from build123d import *

# Parameters (mm, degrees)
SKETCH3_W           = 152.4
SKETCH3_H           = 152.4
BOSS_EXTRUDE1_DEPTH = 12.7
SKETCH5_W           = 147.32
SKETCH5_H           = 7.62
CUT_EXTRUDE1_DEPTH  = 12.7
SKETCH6_W           = 12.7
SKETCH6_H           = 127
CUT_EXTRUDE3_DEPTH  = 12.7
SKETCH8_W           = 7.62
SKETCH8_H           = 7.62
CUT_EXTRUDE4_DEPTH  = 25.4
SKETCH9_W           = 7.62
SKETCH9_H           = 7.62
CUT_EXTRUDE5_DEPTH  = 25.4
SKETCH10_W          = 7.508888552
SKETCH10_H          = 7.62
CUT_EXTRUDE6_DEPTH  = 25.4
SKETCH11_W          = 7.62
SKETCH11_H          = 7.62
BOSS_EXTRUDE3_DEPTH = 25.4
SKETCH12_W          = 7.62
SKETCH12_H          = 7.62
CUT_EXTRUDE7_DEPTH  = 25.4


with BuildPart() as part:
    # Sketch3 → Boss-Extrude1 (new body)
    with BuildSketch(Plane(origin=(0, 0, 0), x_dir=(1, 0, 0), z_dir=(0, 1, 0))):
        with Locations((-76.2, 76.2)):
            Rectangle(SKETCH3_W, SKETCH3_H)
    extrude(amount=BOSS_EXTRUDE1_DEPTH)

    # Sketch5 → Cut-Extrude1 (cut)
    with BuildSketch(Plane.ZY.offset(152.4)):
        with Locations((-76.2, 6.35)):
            Rectangle(SKETCH5_W, SKETCH5_H)
    extrude(amount=-CUT_EXTRUDE1_DEPTH, mode=Mode.SUBTRACT)

    # Sketch6 → Cut-Extrude3 (cut)
    with BuildSketch(Plane(origin=(0, 12.7, 0), x_dir=(1, 0, 0), z_dir=(0, 1, 0))):
        with Locations((-120.65, 76.2)):
            Rectangle(SKETCH6_W, SKETCH6_H)
        with Locations((-95.25, 76.2)):
            Rectangle(SKETCH6_W, SKETCH6_H)
        with Locations((-69.85, 76.2)):
            Rectangle(SKETCH6_W, SKETCH6_H)
        with Locations((-44.45, 76.2)):
            Rectangle(SKETCH6_W, SKETCH6_H)
        with Locations((-19.05, 76.2)):
            Rectangle(SKETCH6_W, SKETCH6_H)
    extrude(amount=-CUT_EXTRUDE3_DEPTH, mode=Mode.SUBTRACT)

    # Sketch8 → Cut-Extrude4 (cut)
    with BuildSketch(Plane(origin=(0, 0, 0), x_dir=(0, 0, -1), z_dir=(1, 0, 0))):
        with Locations((146.05, 6.35)):
            Rectangle(SKETCH8_W, SKETCH8_H)
        with Locations((6.35, 6.35)):
            Rectangle(SKETCH8_W, SKETCH8_H)
    extrude(amount=-CUT_EXTRUDE4_DEPTH, mode=Mode.SUBTRACT)

    # Sketch9 → Cut-Extrude5 (cut)
    with BuildSketch(Plane.XY):
        with Locations((-133.35, 6.35)):
            Rectangle(SKETCH9_W, SKETCH9_H)
    extrude(amount=-CUT_EXTRUDE5_DEPTH, mode=Mode.SUBTRACT)

    # Sketch10 → Cut-Extrude6 (cut)
    with BuildSketch(Plane(origin=(0, 0, -152.4), x_dir=(-1, 0, 0), z_dir=(0, 0, -1))):
        with Locations((133.405555724, 6.35)):
            Rectangle(SKETCH10_W, SKETCH10_H)
    extrude(amount=-CUT_EXTRUDE6_DEPTH, mode=Mode.SUBTRACT)

    # Sketch11 → Boss-Extrude3 (add)
    with BuildSketch(Plane(origin=(-25.4, 0, 0), x_dir=(0, 0, -1), z_dir=(1, 0, 0))):
        with Locations((6.35, 6.35)):
            Rectangle(SKETCH11_W, SKETCH11_H)
    extrude(amount=BOSS_EXTRUDE3_DEPTH)

    # Sketch12 → Cut-Extrude7 (cut)
    with BuildSketch(Plane.XY):
        with Locations((-6.35, 6.35)):
            Rectangle(SKETCH12_W, SKETCH12_H)
    extrude(amount=-CUT_EXTRUDE7_DEPTH, mode=Mode.SUBTRACT)


solid = part.part
Work out the finished part from the listing and answer in its coordinate system (mm). A direction names the side the tool comes from. Give positions to 0.01 mm unless a question says otherwise; leave off trailing zeros. Order: outer loops, then holes, each group sorted by start corner. A loop starts at its lowest first (then second) coordinate and runs counter-clockwise, first axis right, second up. Notation, with made-up numbers: (88, 25.25) -> (113, 25.25) arc R27 ccw to (113, 48.25) -> close; hole circle Ø10 at (-18.5, 12.25). An arc over 180 degrees is marked (long way). One line per item, written item: value.
Item 1: A flat-ended cylindrical pin translates along its axis: P1, Ø2.5, axis at y = 6.5, z = -9.5, coming from the -X side. Find the tip coordinate at first contact, or state that the pin passes through.
Answer sheet:
P1: x = -139.7
Item 2: Find section A-A, the plane z = -132. State how many separate pieces and enclosed holes the cut face has, plus the area to 3 significant figures.
Answer sheet:
separate pieces: 6
enclosed holes: 1
area: 975 mm²
Item 3: Determine the mould class of faces 1 (the flat face through (-13, 6, -149.86)), 2 (the flat face through (-129.651, 6, -140)), 3 (the flat face through (-19, 6, -139.7)) for opening direction X: released by +X, released by -X, zero draft, split by the parting line, or undercut.
Answer sheet:
face 1: zero draft
face 2: undercut
face 3: undercut
Item 4: Straight lines are drawn through the part: probe 1 along X at (y, z) = (7.5, -6); probe 2 along X at (y, z) = (4.25, -87.5); probe 3 along Z at (x, y) = (-120, 3.5). For each, find the intervals that lie inside material, in ascending order.
Answer sheet:
probe 1: -139.7 to -137.16, -129.54 to -10.16, -2.54 to 0
probe 2: -139.7 to -127, -114.3 to -101.6, -88.9 to -76.2, -63.5 to -50.8, -38.1 to -25.4, -12.7 to 0
probe 3: -152.4 to -139.7, -12.7 to 0
Item 5: Find section C-C, the plane z = -91. Give the vertices of the cut face in (x, y), plus the area to 3 significant figures.
Answer sheet:
outline: (-152.4, 0) -> (-127, 0) -> (-127, 12.7) -> (-152.4, 12.7) -> (-152.4, 10.16) -> (-139.7, 10.16) -> (-139.7, 2.54) -> (-152.4, 2.54) -> close; (-114.3, 0) -> (-101.6, 0) -> (-101.6, 12.7) -> (-114.3, 12.7) -> close; (-88.9, 0) -> (-76.2, 0) -> (-76.2, 12.7) -> (-88.9, 12.7) -> close; (-63.5, 0) -> (-50.8, 0) -> (-50.8, 12.7) -> (-63.5, 12.7) -> close; (-38.1, 0) -> (-25.4, 0) -> (-25.4, 12.7) -> (-38.1, 12.7) -> close; (-12.7, 0) -> (0, 0) -> (0, 12.7) -> (-12.7, 12.7) -> close
area: 1,030 mm²
Item 6: Find section B-B, the plane x = -46. Give the vertices of the cut face in (y, z).
Answer sheet:
outline: (0, -152.4) -> (12.7, -152.4) -> (12.7, -139.7) -> (0, -139.7) -> close; (0, -12.7) -> (12.7, -12.7) -> (12.7, 0) -> (0, 0) -> close
Item 7: Find section D-D, the plane x = -132. Give the vertices of the cut face in (y, z).
Answer sheet:
outline: (0, -152.4) -> (2.54, -152.4) -> (2.54, -127) -> (10.16, -127) -> (10.16, -152.4) -> (12.7, -152.4) -> (12.7, 0) -> (10.16, 0) -> (10.16, -25.4) -> (2.54, -25.4) -> (2.54, 0) -> (0, 0) -> close
Item 8: A tool of negligible diameter and unlimited length cuts with its end or side. For faces 4 (the flat face through (-127, 6, -75)), 5 (the flat face through (-146, 2.54, -77)), 6 (the flat face through (-6, 2.54, -13)), from which of +Z, -Z, +X, -X, +Y, -Y can it reach the whole face along a straight path? Write none if from no direction.
Answer sheet:
face 4: +Y, -Y
face 5: -X
face 6: +Z
